Part model, mm, in its own coordinate system. A direction names the side the tool comes from. Give positions to 0.01 mm unless a question says otherwise; leave off trailing zeros. Order: outer loops, then holes, each group sorted by start corner. A loop starts at its lowest first (then second) coordinate and runs counter-clockwise, first axis right, second up. Notation, with made-up numbers: (49, -16) -> (61, -16) arc R18 ccw to (61, 14) -> close; hole circle Ø5 at (61, 21). An arc over 180 degrees is marked (long way). Write item = value, one per line. Start each with the question number.
Item 1: Band-saw the part on A-A on z = 7.5. Write the cut outline in (x, y).
Item 2: Drill centre lines: line 1 along Y through (x, z) = (0, 117.5); line 2 along Z through (x, y) = (-0.15, -0.05). Where is each one in solid material? Low to high.
Item 3: Tool access for faces 1 (the face through (0.748, -0.976, 4.462)), 2 (the face through (0.748, 0.976, 115.538)), 3 (the face through (0, -2.5, 59)): list every direction of +Z, -Z, +X, -X, +Y, -Y with a clear straight run to the whole face (end or side of a thin tool).
Item 4: Flat gauge pin, fed straight in: P1, Ø1.5, axis at x = 0, y = 0, coming from the +Z side. Where does the tip first touch, or does it go through?
Item 5: Pull direction Y, two halves, no side cores. Call faces 4 (the face through (0, 2.5, 59)), 5 (the face through (0.064, 0.204, 9.41)), 6 (the face through (-1, 1, 120)): +Y half, -Y half, draft (parallel to the pull), parting line (faces both ways), or undercut.
Autodesk Inventor part; units mm, degrees
ref_plane "YZ Plane" through (0, 0, 0) normal (1, 0, 0) x (0, 1, 0)
ref_plane "XZ Plane" through (0, 0, 0) normal (0, 1, 0) x (-1, 0, 0)
ref_plane "XY Plane" through (0, 0, 0) normal (0, 0, 1) x (1, 0, 0)
sketch "スケッチ1" plane through (0, 0, 0) normal (0, 0, 1) x (1, 0, 0)
  line L0 (-2.5, 2.5) -> (2.5, 2.5)
  line L1 (2.5, 2.5) -> (2.5, -2.5)
  line L2 (2.5, -2.5) -> (-2.5, -2.5)
  line L3 (-2.5, -2.5) -> (-2.5, 2.5)
  point P0 (0, 0)
  point P1 (-2.5, 0)
  point P2 (0, 2.5)
  dimension "d4" = 5
  dimension "d5" = 5
extrude "押し出し1" add sketch "スケッチ1" along normal blind 120
sketch "スケッチ2" plane through (0, 0, 120) normal (0, 0, 1) x (1, 0, 0)
  point P0 (0, 0)
hole "穴1" at (0, 0, 120) direction (0, 0, -1) diameter 2.459 depth 8.8 tip angle 118
sketch "スケッチ3" plane through (0, 0, 0) normal (0, 0, -1) x (-1, 0, 0)
  point P0 (0, 0)
  point P1 (0, 0)
hole "穴2" at (0, 0, 0) direction (0, 0, 1) diameter 2.459 depth 8.8 tip angle 118
properties part number "回収機構スペーサ"
Values found:
q1.outline = (-2.5, -2.5) -> (2.5, -2.5) -> (2.5, 2.5) -> (-2.5, 2.5) -> close; hole circle Ø2.46 at (0, 0)
q2.line_1 = -2.5 to -1.23, 1.23 to 2.5
q2.line_2 = 9.44 to 110.56
q3.face_1 = -Z
q3.face_2 = +Z
q3.face_3 = +Z, -Z, +X, -X, -Y
q4.P1 = 110.91
q5.face_4 = +Y half
q5.face_5 = undercut
q5.face_6 = draft
